from build123d import *

# Parameters (mm, degrees)
SKETCH10_W            = 156.133449978
SKETCH10_H            = 118.545046658
BOSS_EXTRUDE2_DEPTH   = 3.175
F_5_0MM_DOWEL_HOLE1_D = 5
F_3_0MM_DOWEL_HOLE1_D = 3
F_2_5MM_DOWEL_HOLE1_D = 2.5
F_2_5MM_DOWEL_HOLE2_D = 2.5
F_5_0MM_DOWEL_HOLE2_D = 5


with BuildPart() as part:
    # Sketch10 → Boss-Extrude2 (new body)
    with BuildSketch(Plane.XY):
        with Locations((145.019399685, -105.793370226)):
            Rectangle(SKETCH10_W, SKETCH10_H)
    extrude(amount=BOSS_EXTRUDE2_DEPTH)

    # Ø5.0mm Dowel Hole1 (through all)
    with Locations(Plane.XY.offset(3.175)):
        with Locations((106.452674696, -65.270846897), (186.452674696, -65.270846897), (186.452674696, -145.270846897), (106.452674696, -145.270846897)):
            Hole(F_5_0MM_DOWEL_HOLE1_D / 2)

    # Ø3.0mm Dowel Hole1 (through all)
    with Locations(Plane(origin=(0, 0, 0), x_dir=(-1, 0, 0), z_dir=(0, 0, -1))):
        with Locations((-210.352674696, -58.770846897), (-210.352674696, -151.770846897), (-70.352674696, -154.770846897), (-70.352674696, -59.770846897)):
            Hole(F_3_0MM_DOWEL_HOLE1_D / 2)

    # Ø2.5mm Dowel Hole1 (through all)
    with Locations(Plane(origin=(0, 0, 0), x_dir=(-1, 0, 0), z_dir=(0, 0, -1))):
        with Locations((-200.336124674, -68.770846897), (-83.336124674, -68.770846897), (-83.336124674, -141.770846897), (-200.336124674, -141.770846897)):
            Hole(F_2_5MM_DOWEL_HOLE1_D / 2)

    # Ø2.5mm Dowel Hole2 (through all)
    with Locations(Plane(origin=(0, 0, 0), x_dir=(-1, 0, 0), z_dir=(0, 0, -1))):
        with Locations((-199.336124674, -104.770846897), (-161.336124674, -104.770846897), (-116.036124674, -104.770846897), (-142.336124674, -66.770846897), (-142.336124674, -142.770846897)):
            Hole(F_2_5MM_DOWEL_HOLE2_D / 2)

    # Ø5.0mm Dowel Hole2 (through all)
    with Locations(Plane(origin=(0, 0, 0), x_dir=(-1, 0, 0), z_dir=(0, 0, -1))):
        with Locations((-83.336124674, -105.270846897)):
            Hole(F_5_0MM_DOWEL_HOLE2_D / 2)


solid = part.part
The model under review builds one solid part; all positions refer to its coordinate system, in mm. Round coordinates to 2 decimals unless told otherwise and drop trailing zeros. Answer as a JSON object with one key per item and string values.
1. Clearance check with flat-ended pins moving along their axes: pin 1 (5 mm diameter, centred on x = 210.35, y = -151.77, fed in from -Z); pin 2 (1.5 mm diameter, centred on x = 199.34, y = -104.77, fed in from -Z). State where each tip first meets the part, or that it passes through.
Results found:
{"pin 1": "stops at z = 0", "pin 2": "passes through"}
2. The part is to be moulded in two halves that separate along Y. For faces 1 (the face through (144, -165.066, 2)), 2 (the face through (184.07, -144.52, 1.57)), 3 (the face through (66.953, -107, 2)), say which applies: pulls with the +Y half, pulls with the -Y half, needs draft (parallel to the pull), parting line crosses it, or undercut.
Results found:
{"face 1": "pulls with the -Y half", "face 2": "undercut", "face 3": "needs draft"}
3. To check wall thickness, follow line 1 along Y through (x, z) = (142.5, 2); line 2 along Y through (x, z) = (161.5, 3); line 3 along X through (y, z) = (-151.5, 0.9). State the ranges of each line that lie inside material, in increasing order.
Results found:
{"line 1": "y = -165.07 to -144.01, -141.53 to -68.01, -65.53 to -46.52", "line 2": "y = -165.07 to -106.01, -103.53 to -46.52", "line 3": "x = 66.95 to 208.88, 211.83 to 223.09"}
